```python
from build123d import *

# Parameters (mm, degrees)
F1_DEPTH = 25


with BuildPart() as f1:
    # F0 (on Front) → F1 (new body)
    with BuildSketch(Plane.XZ):
        with BuildLine():
            Line((-349.718489, 37.126835), (194.89311, 37.126835))
            Line((194.89311, 37.126835), (-199.541794, 253.739637))
            Line((-199.541794, 253.739637), (-199.541794, 303.739637))
            Line((-199.541794, 303.739637), (-127.248838, 447.979555))
            ThreePointArc((-127.248838, 447.979555), (-119.334756, 469.764715), (-116.648626, 492.786673))
            Line((-116.648626, 492.786673), (-116.648626, 840.545695))
            ThreePointArc((-116.648626, 840.545695), (-131.553761, 893.070584), (-171.825906, 929.937661))
            Line((-171.825906, 929.937661), (-326.719748, 1007.604186))
            Line((-326.719748, 1007.604186), (-397.71723, 1007.604186))
            Line((-397.71723, 1007.604186), (-552.611073, 929.937661))
            ThreePointArc((-552.611073, 929.937661), (-592.883217, 893.070584), (-607.788352, 840.545695))
            Line((-607.788352, 840.545695), (-607.788352, 492.786673))
            ThreePointArc((-607.788352, 492.786673), (-605.102223, 469.764715), (-597.188141, 447.979555))
            Line((-597.188141, 447.979555), (-524.895184, 303.739637))
            Line((-524.895184, 303.739637), (-524.895184, 253.739637))
            Line((-524.895184, 253.739637), (-919.330089, 37.126835))
            Line((-919.330089, 37.126835), (-374.718489, 37.126835))
            Line((-374.718489, 37.126835), (-374.718489, 522.281469))
            ThreePointArc((-374.718489, 522.281469), (-374.718772, 522.365511), (-374.718489, 522.449553))
            ThreePointArc((-374.718489, 522.449553), (-362.218489, 534.865793), (-349.718489, 522.449553))
            ThreePointArc((-349.718489, 522.449553), (-349.718207, 522.365511), (-349.718489, 522.281469))
            Line((-349.718489, 522.281469), (-349.718489, 37.126835))
        make_face()
        with BuildLine():
            Line((-349.718489, 522.449553), (-349.718489, 522.281469))
            ThreePointArc((-349.718489, 522.281469), (-349.718207, 522.365511), (-349.718489, 522.449553))
        make_face()
        with BuildLine():
            Line((-374.718489, 522.281469), (-374.718489, 522.449553))
            ThreePointArc((-374.718489, 522.449553), (-374.718772, 522.365511), (-374.718489, 522.281469))
        make_face()
    extrude(amount=F1_DEPTH)


solid = f1.part
```
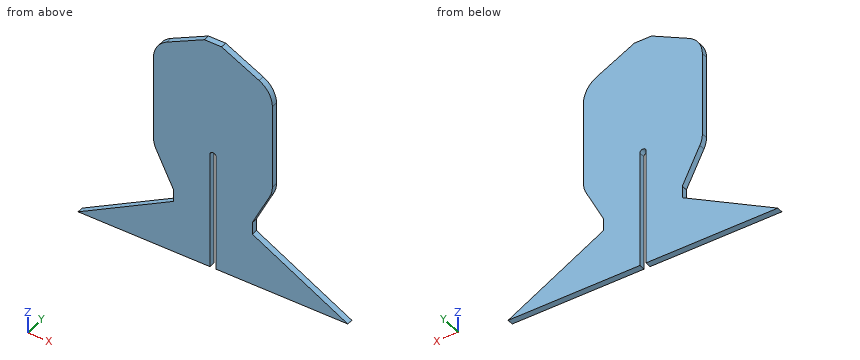
Part model, mm, in its own coordinate system. Coordinates: 2 decimals unless noted, no trailing zeros. Order: outer loops, then holes, each group sorted by start corner. A loop starts at its lowest first (then second) coordinate and runs counter-clockwise, first axis right, second up. Notation, with made-up numbers: (60.5, 63) - (68.5, 63) arc R29 ccw to (68.5, 102) - close; hole circle Ø7 at (58.5, 25.5). An arc over 180 degrees is marked (long way). Return JSON: item names as keys, results as strings. Group by question number.
Item 1: Cut at D-D (z = 142.5). List the corners of the cut face in (x, y), plus the area to 3 significant figures.
Item 2: Cut at C-C (z = 620). List the corners of the cut face in (x, y).
Item 3: Pin check, flat tips, straight feed: pin 1 (1 mm diameter, centred on x = -770.5, y = -9, fed in from +Z); pin 2 (4 mm diameter, centred on y = -7.5, z = 558, fed in from -X); pin 3 (12.5 mm diameter, centred on y = -6.5, z = 223.5, fed in from +X). Stop position of each tip, or through.
Item 4: Cut at B-B (y = -20.25). List the corners of the cut face in (x, z), plus the area to 3 significant figures.
Item 5: Cut at A-A (z = 289.5). List the corners of the cut face in (x, y), plus the area to 3 significant figures.
Item 6: Drill centre lines: probe 1 along X at (y, z) = (-11, 492); probe 2 along X at (y, z) = (-2.25, 295); probe 3 along X at (y, z) = (-15, 589.5). Where is each one in solid material? Low to high. Write a range as from..to.
Check values:
{
 "1": {"outline": "(-727.45, -25) - (-374.72, -25) - (-374.72, 0) - (-727.45, 0) - close; (-349.72, -25) - (3.02, -25) - (3.02, 0) - (-349.72, 0) - close", "area": "17,600 mm2"},
 "2": {"outline": "(-607.79, -25) - (-116.65, -25) - (-116.65, 0) - (-607.79, 0) - close"},
 "3": {"pin 1": "stops at z = 119.13", "pin 2": "stops at x = -607.79", "pin 3": "stops at x = -133.1"},
 "4": {"outline": "(-919.33, 37.13) - (-374.72, 37.13) - (-374.72, 522.45) arc R12.5 cw to (-349.72, 522.45) - (-349.72, 37.13) - (194.89, 37.13) - (-199.54, 253.74) - (-199.54, 303.74) - (-127.25, 447.98) arc R100 ccw to (-116.65, 492.79) - (-116.65, 840.55) arc R100 ccw to (-171.83, 929.94) - (-326.72, 1007.6) - (-397.72, 1007.6) - (-552.61, 929.94) arc R100 ccw to (-607.79, 840.55) - (-607.79, 492.79) arc R100 ccw to (-597.19, 447.98) - (-524.9, 303.74) - (-524.9, 253.74) - close", "area": "468,000 mm2"},
 "5": {"outline": "(-524.9, -25) - (-374.72, -25) - (-374.72, 0) - (-524.9, 0) - close; (-349.72, -25) - (-199.54, -25) - (-199.54, 0) - (-349.72, 0) - close", "area": "7,510 mm2"},
 "6": {"probe 1": "x = -607.79..-374.72, -349.72..-116.65", "probe 2": "x = -524.9..-374.72, -349.72..-199.54", "probe 3": "x = -607.79..-116.65"}
}
